CAD build for the part. Positions are in the model's coordinates, mm. Round coordinates to 2 decimals unless told otherwise and drop trailing zeros. Order: outer loops, then holes, each group sorted by start corner. A loop starts at its lowest first (then second) coordinate and runs counter-clockwise, first axis right, second up. Notation, with made-up numbers: M -21.75,2.25 L -0.75,2.25 A20 ccw -0.75,26.25 Z; hole C 25,49.25 d9. An arc over 180 degrees is marked long. Answer as a JSON object with one key per item and string values.
```python
from build123d import *

# Parameters (mm, degrees)
F0_W     = 1143
F0_H     = 558.8
F1_DEPTH = 101.6
F3_DEPTH = 101.6


with BuildPart() as f1:
    # F0 (on Front) → F1 (new body)
    with BuildSketch(Plane.XZ):
        Rectangle(F0_W, F0_H)
    extrude(amount=F1_DEPTH)

    # F2 (on face) → F3 (join)
    with BuildSketch(Plane.XZ.offset(101.6)):
        with BuildLine():
            Line((0, 0), (49.957755, 0))
            ThreePointArc((49.957755, 0), (35.325468, 35.325468), (0, 49.957755))
            Line((0, 49.957755), (0, 0))
        make_face()
        with BuildLine():
            ThreePointArc((0, -49.957755), (35.325468, -35.325468), (49.957755, 0))
            Line((49.957755, 0), (0, 0))
            Line((0, 0), (0, -49.957755))
        make_face()
        with BuildLine():
            Line((0, 0), (0, 49.957755))
            ThreePointArc((0, 49.957755), (-35.325468, 35.325468), (-49.957755, 0))
            Line((-49.957755, 0), (0, 0))
        make_face()
        with BuildLine():
            ThreePointArc((-49.957755, 0), (-35.325468, -35.325468), (0, -49.957755))
            Line((0, -49.957755), (0, 0))
            Line((0, 0), (-49.957755, 0))
        make_face()
    extrude(amount=F3_DEPTH)


solid = f1.part
```
Item 1: Saw through at B-B on z = -210.5. List the corners of the cut face in (x, y), and give its area (3 significant figures).
Worked answers:
{"outline": "M -571.5,-101.6 L 571.5,-101.6 L 571.5,0 L -571.5,0 Z", "area": "116,000 mm2"}
Item 2: Wall check: line 1 along Y through (x, z) = (488.5, -199); line 2 along X through (y, z) = (-150, 5); line 3 along X through (y, z) = (-130.5, -4.5). Give the ranges that are in metal, low to high. Write a range as [from, to].
Worked answers:
{"line 1": "y = [-101.6, 0]", "line 2": "x = [-49.71, 49.71]", "line 3": "x = [-49.75, 49.75]"}
Item 3: Saw through at C-C on x = 25. List the corners of the cut face in (y, z), and give its area (3 significant figures).
Worked answers:
{"outline": "M -203.2,-43.25 L -101.6,-43.25 L -101.6,-279.4 L 0,-279.4 L 0,279.4 L -101.6,279.4 L -101.6,43.25 L -203.2,43.25 Z", "area": "65,600 mm2"}
Item 4: Saw through at A-A on y = -182.5. List the corners of the cut face in (x, z), and give its area (3 significant figures).
Worked answers:
{"outline": "M -49.96,0 A49.96 ccw 0,-49.96 A49.96 ccw 49.96,0 A49.96 ccw 0,49.96 A49.96 ccw Z", "area": "7,840 mm2"}
Item 5: Drop a flat-ended pin along its axis: pin 1 Ø10 at (x, z) = (-112.5, 53.5) entering from -Y. Give the stop position or say it passes through.
Worked answers:
{"pin 1": "stops at y = -101.6"}
